The listing builds one solid part. Answer for the finished solid, in the listing's coordinates (mm). A direction names the side the tool comes from. Round coordinates to 2 decimals unless told otherwise and drop trailing zeros. Order: outer loops, then holes, each group sorted by start corner. A loop starts at its lowest first (then second) coordinate and runs counter-clockwise, first axis right, second up. Notation, with made-up numbers: (75.5, 63) - (115.5, 63) arc R32 cw to (115.5, 90) - close; hole circle Ø8 at (2, 29). An arc over 180 degrees is marked (long way). Write item = value, one per line.
from build123d import *

# Parameters (mm, degrees)
HOLE_WIZARD_M3_1_D = 2.5
HOLE_WIZARD_M5_1_D = 4.2
CHAMFER_1_SIZE     = 0.5


with BuildPart() as part:
    # 草图1 → 旋转1 (revolve)
    with BuildSketch(Plane.XY):
        Polygon((0, 8), (0, 0), (3, 0), (3, -0.9), (4, -0.9), (4, 0), (11, 0), (11, 4), (4, 4), (4, 8), align=None)
    revolve(axis=Axis((0, 0, 0), (0, -1, 0)))

    # M3 螺纹孔1 (through all)
    with Locations(Plane(origin=(0, 4, 0), x_dir=(1, 0, 0), z_dir=(0, 1, 0))):
        with Locations((-6.495190528, 3.75), (6.495190528, 3.75), (0, -7.5)):
            Hole(HOLE_WIZARD_M3_1_D / 2)

    # M5 螺纹孔1 (through all)
    with Locations(Plane(origin=(0, 0, 0), x_dir=(-1, 0, 0), z_dir=(0, -1, 0))):
        with Locations((0, 0)):
            Hole(HOLE_WIZARD_M5_1_D / 2)

    # 倒角1
    chamfer_1_edges = [part.edges().sort_by_distance(p)[0] for p in [
        (-4, 8, 0),
        (-11, 4, 0),
        (-11, 0, 0),
        (-4, 0, 0),
    ]]
    chamfer(chamfer_1_edges, length=CHAMFER_1_SIZE)


solid = part.part
Q1. For faces 4 (the face through (2.003, 4.056, -0.631)), 5 (the face through (-3, -0.5, 0.1)), 6 (the face through (5, 4, 0)), determine the directions among +Z, -Z, +X, -X, +Y, -Y from which every point of the face is accessible in a straight line to the end or side of a thin tool.
Model answer:
face_4 = +Y, -Y
face_5 = -Y
face_6 = +Y
Q2. Find the intervals of material crossed by line 1 (Z direction, x = 0, y = 3.25); line 2 (X direction, y = 1, z = -3.5); line 3 (Y direction, x = -9, z = -1), in increasing order. Write a range as from..to.
Model answer:
line_1 = -11..-2.1, 2.1..6.25, 8.75..11
line_2 = -10.43..-7.72, -5.27..5.27, 7.72..10.43
line_3 = 0..4
Q3. Determine the mould class of faces 1 (the face through (2, 8, -2)), 2 (the face through (-2.38, 2.02, -10.74)), 3 (the face through (0.27, 1.97, 8.72)) for opening direction Z: released by +Z, released by -Z, zero draft, split by the parting line, or undercut.
Model answer:
face_1 = zero draft
face_2 = split by the parting line
face_3 = undercut
Q4. Section C-C on y = 3 is taken. Determine the outline of the cut face in (x, z).
Model answer:
outline = circle Ø22 at (0, 0); hole circle Ø2.5 at (-6.5, -3.75); hole circle Ø4.2 at (0, 0); hole circle Ø2.5 at (0, 7.5); hole circle Ø2.5 at (6.5, -3.75)
Q5. Section D-D on y = 5 is taken. Determine the outline of the cut face in (x, z).
Model answer:
outline = circle Ø8 at (0, 0); hole circle Ø4.2 at (0, 0)
Q6. Section A-A on z = 0 is taken. Determine the outline of the cut face in (x, y).
Model answer:
outline = (-11, 0.5) - (-10.5, 0) - (-4.5, 0) - (-4, -0.5) - (-4, -0.9) - (-3, -0.9) - (-3, 0) - (-2.1, 0) - (-2.1, 8) - (-3.5, 8) - (-4, 7.5) - (-4, 4) - (-10.5, 4) - (-11, 3.5) - close; (2.1, 0) - (3, 0) - (3, -0.9) - (4, -0.9) - (4, -0.5) - (4.5, 0) - (10.5, 0) - (11, 0.5) - (11, 3.5) - (10.5, 4) - (4, 4) - (4, 7.5) - (3.5, 8) - (2.1, 8) - close
Q7. Section B-B on x = 0 is taken. Count the separate pieces of the cut face and the enclosed holes in it, then the cut area to 3 significant figures.
Model answer:
separate_pieces = 3
enclosed_holes = 0
area = 77.7 mm^2
Q8. Flat-ended cylindrical pins translate along their axes: P1, Ø4, axis at x = 0, z = 7.5, coming from the -Y side; P2, Ø2, axis at y = 5.5, z = 0, coming from the -X side; P3, Ø1.5, axis at x = 0, y = 6.5, coming from the -Z side; P4, Ø3.5, axis at x = 0, z = 0, coming from the -Y side. Find the tip coordinate at first contact, or state that the pin passes through.
Model answer:
P1 = 0
P2 = -4
P3 = -4
P4 = through
